```python
from build123d import *

# Parameters (mm, degrees)
SALIENTE_EXTRUIR1_DEPTH             = 2.5
CROQUIS2_W                          = 51
CROQUIS2_H                          = 2.5
SALIENTE_EXTRUIR2_DEPTH             = 36.177083333
SALIENTE_EXTRUIR3_DEPTH             = 2.5
CROQUIS4_W                          = 51.5
CROQUIS4_H                          = 2.5
SALIENTE_EXTRUIR4_DEPTH             = 9
CORTAR_EXTRUIR1_DEPTH               = 122.155458756
DI_METRO_DE_TALADRO_5_1_5_1_1_D     = 5.1
DI_METRO_DE_TALADRO_5_1_5_1_1_DEPTH = 53.5
DI_METRO_DE_TALADRO_5_1_5_1_2_D     = 5.1
DI_METRO_DE_TALADRO_7_2_7_2_1_D     = 7.2
DI_METRO_DE_TALADRO_23_0_23_1_D     = 23
DI_METRO_DE_TALADRO_23_0_23_1_DEPTH = 9.015002711
DI_METRO_DE_TALADRO_3_5_3_5_1_D     = 3.5
DI_METRO_DE_TALADRO_3_5_3_5_1_DEPTH = 9.015002711
REDONDEO1_R                         = 2
REDONDEO2_R                         = 5
REDONDEO3_R                         = 8
REDONDEO4_R                         = 11.5
REDONDEO5_R                         = 12
CORTAR_EXTRUIR2_DEPTH               = 10


with BuildPart() as part:
    # Croquis1 → Saliente-Extruir1 (new body)
    with BuildSketch(Plane(origin=(0, 43.526431985, 0), x_dir=(1, 0, 0), z_dir=(0, 1, 0))):
        Polygon((24.760416667, 29.4), (51.322916667, 29.4), (51.322916667, 80.4), align=None)
    extrude(amount=-SALIENTE_EXTRUIR1_DEPTH)

    # Croquis2 → Saliente-Extruir2 (add)
    with BuildSketch(Plane(origin=(51.322916667, 0, 0), x_dir=(0, 0, -1), z_dir=(1, 0, 0))):
        with Locations((54.9, 42.276431985)):
            Rectangle(CROQUIS2_W, CROQUIS2_H)
    extrude(amount=SALIENTE_EXTRUIR2_DEPTH)

    # Croquis3 → Saliente-Extruir3 (add)
    with BuildSketch(Plane.XY.offset(-29.4)):
        Polygon((0, -38.607215424), (0, 38.4885797), (14.488727812, 50.041434696), (25.5, 43.526431985), (87.5, 43.526431985), (87.5, -6.900242064), (14.886977722, -49.162809247), align=None)
    extrude(amount=SALIENTE_EXTRUIR3_DEPTH)

    # Croquis4 → Saliente-Extruir4 (add)
    with BuildSketch(Plane(origin=(87.5, 0, 0), x_dir=(0, 0, -1), z_dir=(1, 0, 0))):
        with Locations((54.65, 42.276431985)):
            Rectangle(CROQUIS4_W, CROQUIS4_H)
    extrude(amount=SALIENTE_EXTRUIR4_DEPTH)

    # Croquis5 → Cortar-Extruir1 (cut, through all)
    with BuildSketch(Plane.XY.offset(-26.9)):
        Polygon((0, 22.5), (0, -35.5), (9, -35.5), (9, -22.5), (22.5, -22.5), (22.5, 22.5), align=None)
    extrude(amount=-CORTAR_EXTRUIR1_DEPTH, mode=Mode.SUBTRACT)

    # Diámetro de taladro Ø5.1 (5.1)1
    with Locations(Plane.XY.offset(-26.9)):
        with Locations((56, 0), (30, 0)):
            Hole(DI_METRO_DE_TALADRO_5_1_5_1_1_D / 2, depth=DI_METRO_DE_TALADRO_5_1_5_1_1_DEPTH)

    # Diámetro de taladro Ø5.1 (5.1)2 (through all)
    with Locations(Plane(origin=(0, 0, -29.4), x_dir=(-1, 0, 0), z_dir=(0, 0, -1))):
        with Locations((-15.4, -35.5), (-15.4, 35.5)):
            Hole(DI_METRO_DE_TALADRO_5_1_5_1_2_D / 2)

    # Diámetro de taladro Ø7.2 (7.2)1 (through all)
    with Locations(Plane(origin=(0, 0, -29.4), x_dir=(-1, 0, 0), z_dir=(0, 0, -1))):
        with Locations((-75.6, 0)):
            Hole(DI_METRO_DE_TALADRO_7_2_7_2_1_D / 2)

    # Diámetro de taladro Ø23.0 (23)1
    with Locations(Plane(origin=(0, 41.026431985, 0), x_dir=(-1, 0, 0), z_dir=(0, -1, 0))):
        with Locations((-75.5, 59.4)):
            Hole(DI_METRO_DE_TALADRO_23_0_23_1_D / 2, depth=DI_METRO_DE_TALADRO_23_0_23_1_DEPTH)

    # Diámetro de taladro Ø3.5 (3.5)1
    with Locations(Plane(origin=(0, 41.026431985, 0), x_dir=(-1, 0, 0), z_dir=(0, -1, 0))):
        with Locations((-60, 74.9), (-91, 43.9), (-60, 43.9), (-91, 74.9)):
            Hole(DI_METRO_DE_TALADRO_3_5_3_5_1_D / 2, depth=DI_METRO_DE_TALADRO_3_5_3_5_1_DEPTH)

    # Redondeo1
    redondeo1_edges = [part.edges().sort_by_distance(p)[0] for p in [
        (0, -38.607215424, -28.15),
        (0, 38.4885797, -28.15),
        (0, 22.5, -28.15),
        (22.5, 22.5, -28.15),
        (22.5, -22.5, -28.15),
        (9, -22.5, -28.15),
        (9, -35.5, -28.15),
        (0, -35.5, -28.15),
    ]]
    fillet(redondeo1_edges, radius=REDONDEO1_R)

    # Redondeo2
    redondeo2_edges = [part.edges().sort_by_distance(p)[0] for p in [
        (96.5, 42.276431985, -80.4),
        (51.322916667, 42.276431985, -80.4),
    ]]
    fillet(redondeo2_edges, radius=REDONDEO2_R)

    # Redondeo3
    redondeo3_edges = [part.edges().sort_by_distance(p)[0] for p in [
        (25.5, 43.526431985, -28.15),
        (96.5, 42.276431985, -28.9),
    ]]
    fillet(redondeo3_edges, radius=REDONDEO3_R)

    # Redondeo4
    redondeo4_edges = [part.edges().sort_by_distance(p)[0] for p in [
        (14.886977722, -49.162809247, -28.15),
    ]]
    fillet(redondeo4_edges, radius=REDONDEO4_R)

    # Redondeo5
    redondeo5_edges = [part.edges().sort_by_distance(p)[0] for p in [
        (87.5, -6.900242064, -28.15),
        (14.488727812, 50.041434696, -28.15),
    ]]
    fillet(redondeo5_edges, radius=REDONDEO5_R)

    # Croquis19 → Cortar-Extruir2 (cut)
    with BuildSketch(Plane(origin=(0, 43.526431985, 0), x_dir=(1, 0, 0), z_dir=(0, 1, 0))):
        with BuildLine():
            Line((42.255993265, 44.007837327), (42.270997317, 45.507687231))
            ThreePointArc((42.270997317, 45.507687231), (47.390937401, 50.576665136), (52.510877484, 45.507687231))
            Line((52.510877484, 45.507687231), (52.525881536, 44.007837327))
            ThreePointArc((52.525881536, 44.007837327), (47.390937401, 38.821267806), (42.255993265, 44.007837327))
        make_face()
        with BuildLine():
            Line((45.903627778, 34.856468872), (45.903627778, 36.556468872))
            ThreePointArc((45.903627778, 36.556468872), (47.390937401, 38.043778494), (48.878247023, 36.556468872))
            Line((48.878247023, 36.556468872), (48.878247023, 34.856468872))
            ThreePointArc((48.878247023, 34.856468872), (47.390937401, 33.36915925), (45.903627778, 34.856468872))
        make_face()
        with BuildLine():
            Line((45.898554991, 52.856468872), (45.898554991, 54.556468872))
            ThreePointArc((45.898554991, 54.556468872), (47.390937401, 56.048851282), (48.883319811, 54.556468872))
            Line((48.883319811, 54.556468872), (48.883319811, 52.856468872))
            ThreePointArc((48.883319811, 52.856468872), (47.390937401, 51.364086462), (45.898554991, 52.856468872))
        make_face()
    extrude(amount=-CORTAR_EXTRUIR2_DEPTH, mode=Mode.SUBTRACT)


solid = part.part
```
Source: CAD feature listing. Evaluate the final solid. Frame: model axes, mm. A direction names the side the tool comes from. Coordinates: 2 decimals unless noted, no trailing zeros. Loops run counter-clockwise (first coordinate to the right, second up) from the corner with the lowest first, then second, coordinate; pieces in that order, holes last. Notation, with made-up numbers: M 24.25,55 L 42.25,55 A12 cw 42.25,74 Z; hole C -20,-33 d11. An arc over 180 degrees is marked long. Put each result on its own line as item: value. Start each with the question number.
1) Reachability of faces 1 (the face through (4, -35.5, -28)), 2 (the face through (47.505, 42.294, -38.823)), 3 (the face through (73, 42, -80.4)) from +Z, -Z, +X, -X, +Y, -Y: full face, straight path, thin tool, end or side. Return the list, or none.
2) Ray query, L1, parallel to Z at x = 60, y = 42; L2, parallel to Y at x = 86.5, z = -54; L3, parallel to Z at x = 30.5, y = -35. Return the intervals inside material, ascending. Write a range as from..to.
3) Cut plane B-B on z = -59.4. Return the cut outline in (x, y), then the cut area to 3 significant figures.
4) Contact query for flat-ended pins moving along their axis: pin 1 Ø1.5 at (x, y) = (77, 13) entering from -Z; pin 2 Ø0.8 at (x, z) = (14.5, -28) entering from +Y (3 decimals); pin 3 Ø1 at (x, z) = (62, -51.5) entering from +Y; pin 4 Ø14 at (x, z) = (75.5, -59.4) entering from +Y. Output: stop coordinate, or through.
5) Cut plane C-C on x = 29.5. Return the cut outline in (y, z).
6) Pull-direction query (Y, two-part tool) for faces 4 (the face through (9, -29, -28)), 5 (the face through (4.9, -42.08, -28.17)), 6 (the face through (77.261, -3.194, -28.132)), 7 (the face through (87.5, 22, -28)); classes: pulls with the +Y half, pulls with the -Y half, needs draft (parallel to the pull), parting line crosses it, or undercut.
7) Cut plane D-D on x = 15.4. Return the cut outline in (y, z), then the cut area to 3 significant figures.
8) Cut plane A-A on x = 75.6. Return the cut outline in (y, z), then the cut area to 3 significant figures.
The answers:
1. face 1: +Z, -Z, -X
1. face 2: +Y, -Y
1. face 3: -Z, +X, -X, +Y, -Y
2. L1: z = -80.4..-76.65, -73.15..-45.65, -42.15..-26.9
2. L2: y = 41.03..43.53
2. L3: z = -29.4..-26.9
3. outline: M 40.39,41.03 L 64,41.03 L 64,43.53 L 40.39,43.53 Z; M 87,41.03 L 96.5,41.03 L 96.5,43.53 L 87,43.53 Z
3. area: 82.8 mm²
4. pin 1: stops at z = -29.4
4. pin 2: stops at y = 47.485
4. pin 3: stops at y = 43.53
4. pin 4: passes through
5. outline: M -40.66,-29.4 L -2.5,-29.4 L -2.5,-26.9 L -40.66,-26.9 Z; M 2.5,-29.4 L 41.03,-29.4 L 41.03,-38.5 L 43.53,-38.5 L 43.53,-26.9 L 2.5,-26.9 Z
6. face 4: undercut
6. face 5: pulls with the -Y half
6. face 6: undercut
6. face 7: needs draft
7. outline: M -47,-29.4 L -38.05,-29.4 L -38.05,-26.9 L -47,-26.9 Z; M -32.95,-29.4 L -22.5,-29.4 L -22.5,-26.9 L -32.95,-26.9 Z; M 22.5,-29.4 L 32.95,-29.4 L 32.95,-26.9 L 22.5,-26.9 Z; M 38.05,-29.4 L 47.5,-29.4 L 47.5,-26.9 L 38.05,-26.9 Z
7. area: 98.2 mm²
8. outline: M -13.83,-29.4 L -3.6,-29.4 L -3.6,-26.9 L -13.83,-26.9 Z; M 3.6,-29.4 L 41.03,-29.4 L 41.03,-47.9 L 43.53,-47.9 L 43.53,-26.9 L 3.6,-26.9 Z; M 41.03,-80.4 L 43.53,-80.4 L 43.53,-70.9 L 41.03,-70.9 Z
8. area: 195 mm²
